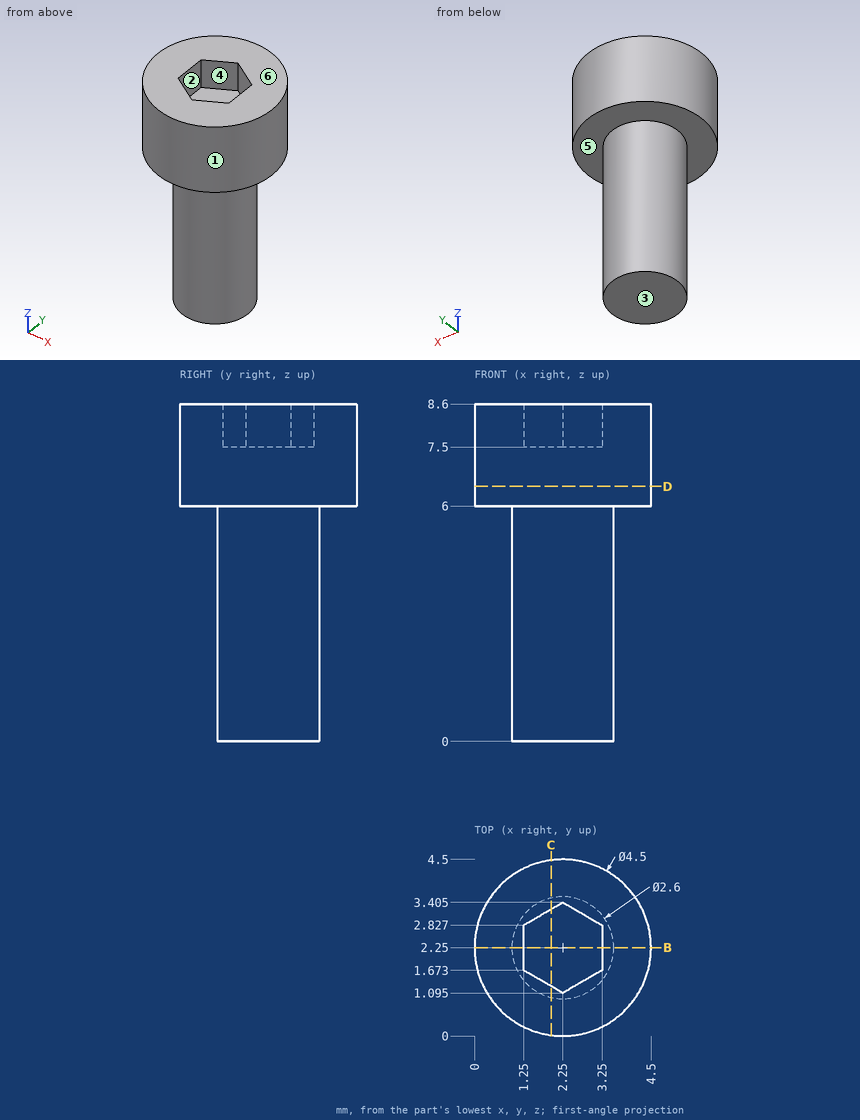
Design review of the part shown in the three views and the two pictorial views. Dimensions are in mm from the part's minimum x, y and z. A direction names the side the tool comes from. Round coordinates to 2 decimals unless told otherwise and drop trailing zeros. Write each loop counter-clockwise with the first axis right and the second up, starting at its lowest first coordinate (ties: lowest second). Pieces come first, ordered by that corner, then holes.
1) Machinability: for the marked faces 5 and 6, which of the approach directions +Z, -Z, +X, -X, +Y, -Y give a long, thin tool a straight path to every point of the face, cutting with its end or side? Answer none if there is none.
Answer below:
face 5: -Z
face 6: +Z, +X, -X, +Y, -Y
2) Take a section at B-B on y = 2.25. Give the boundary of the cut face in (x, z), then the cut area to 3 significant figures.
Answer below:
outline: (0, 6) - (0.95, 6) - (0.95, 0) - (3.55, 0) - (3.55, 6) - (4.5, 6) - (4.5, 8.6) - (3.25, 8.6) - (3.25, 7.5) - (1.25, 7.5) - (1.25, 8.6) - (0, 8.6) - close
area: 25.1 mm2
3) Insertion check: pin 1 Ø2 at (x, z) = (4, 2.5) entering from +Y; pin 2 Ø1 at (x, y) = (2, 2.5) entering from +Z; pin 3 Ø2 at (y, z) = (2, 4) entering from +X. Each pin has a flat end and moves straight along its axis. Give the tip position at first contact, or say it passes through.
Answer below:
pin 1: stops at y = 3.31
pin 2: stops at z = 7.5
pin 3: stops at x = 3.55
4) Mouldability with a two-part tool opening along Y and no side actions: class the marked faces 1, 2, 3 and 4 as +Y half, -Y half, draft (parallel to the pull), parting line (faces both ways), or undercut.
Answer below:
face 1: parting line
face 2: undercut
face 3: draft
face 4: undercut
5) Take a section at C-C on x = 1.95. Give the boundary of the cut face in (y, z) (1 decimal), then the cut area to 3 significant figures.
Answer below:
outline: (0, 6) - (1, 6) - (1, 0) - (3.5, 0) - (3.5, 6) - (4.5, 6) - (4.5, 8.6) - (3.2, 8.6) - (3.2, 7.5) - (1.3, 7.5) - (1.3, 8.6) - (0, 8.6) - close
area: 24.6 mm2
6) Take a section at D-D on z = 6.5. Give the boundary of the cut face in (x, y).
Answer below:
outline: circle Ø4.5 at (2.25, 2.25)
7) For line 1 along Z through (x, y) = (2.15, 2.8); line 2 along Z through (x, y) = (3.7, 2.4); line 3 along X through (y, z) = (3.2, 8) (1 decimal), list the stretches that pass through material, from the lowest coordinate up.
Answer below:
line 1: z = 0 to 7.5
line 2: z = 6 to 8.6
line 3: x = 0.2 to 1.9, 2.6 to 4.3
